Build history of the part. All positions in model axes, mm. Coordinates: 2 decimals unless noted, no trailing zeros. Order: outer loops, then holes, each group sorted by start corner. A loop starts at its lowest first (then second) coordinate and runs counter-clockwise, first axis right, second up. Notation, with made-up numbers: (11.5, 22) - (60.5, 22) arc R15 ccw to (60.5, 47) - close; hole circle Ø3 at (35, 9). An arc over 180 degrees is marked (long way). One line per item, written item: value.
from build123d import *

# Parameters (mm, degrees)
MODEL_R         = 1.5
MODEL_R_2       = 3.25
MODEL_R_3       = 1.25
EXTRUDE_1_DEPTH = 1


with BuildPart() as part:
    # Model → Бобышка-Вытянуть1 (new body)
    with BuildSketch(Plane.XY):
        with BuildLine():
            Line((-28.5, -69), (28.5, -69))
            ThreePointArc((28.5, -69), (29.207106781, -68.707106781), (29.5, -68))
            Line((29.5, -68), (29.5, -61))
            ThreePointArc((29.5, -61), (29.792893219, -60.292893219), (30.5, -60))
            Line((30.5, -60), (39, -60))
            ThreePointArc((39, -60), (39.707106781, -59.707106781), (40, -59))
            Line((40, -59), (40, -55))
            Line((40, -55), (40, -51))
            ThreePointArc((40, -51), (39.707106781, -50.292893219), (39, -50))
            Line((39, -50), (30.5, -50))
            ThreePointArc((30.5, -50), (29.792893219, -49.707106781), (29.5, -49))
            Line((29.5, -49), (29.5, -11))
            ThreePointArc((29.5, -11), (29.792893219, -10.292893219), (30.5, -10))
            Line((30.5, -10), (39, -10))
            ThreePointArc((39, -10), (39.707106781, -9.707106781), (40, -9))
            Line((40, -9), (40, -5))
            Line((40, -5), (40, -1))
            ThreePointArc((40, -1), (39.707106781, -0.292893219), (39, 0))
            Line((39, 0), (30.5, 0))
            ThreePointArc((30.5, 0), (29.792893219, 0.292893219), (29.5, 1))
            Line((29.5, 1), (29.5, 18))
            ThreePointArc((29.5, 18), (29.207106781, 18.707106781), (28.5, 19))
            Line((28.5, 19), (-28.5, 19))
            ThreePointArc((-28.5, 19), (-29.207106781, 18.707106781), (-29.5, 18))
            Line((-29.5, 18), (-29.5, 1))
            ThreePointArc((-29.5, 1), (-29.792893219, 0.292893219), (-30.5, 0))
            Line((-30.5, 0), (-39, 0))
            ThreePointArc((-39, 0), (-39.707106781, -0.292893219), (-40, -1))
            Line((-40, -1), (-40, -5))
            Line((-40, -5), (-40, -9))
            Line((-40, -9), (-40, -52))
            Line((-40, -52), (-40, -55))
            Line((-40, -55), (-40, -59))
            ThreePointArc((-40, -59), (-39.707106781, -59.707106781), (-39, -60))
            Line((-39, -60), (-30.5, -60))
            ThreePointArc((-30.5, -60), (-29.792893219, -60.292893219), (-29.5, -61))
            Line((-29.5, -61), (-29.5, -68))
            ThreePointArc((-29.5, -68), (-29.207106781, -68.707106781), (-28.5, -69))
        make_face()
        with Locations((-35, -5)):
            Circle(MODEL_R, mode=Mode.SUBTRACT)
        with Locations((-35, -55)):
            Circle(MODEL_R, mode=Mode.SUBTRACT)
        with Locations((35, -5)):
            Circle(MODEL_R, mode=Mode.SUBTRACT)
        with Locations((35, -55)):
            Circle(MODEL_R, mode=Mode.SUBTRACT)
        with Locations((-34, -20.4)):
            Circle(MODEL_R_2, mode=Mode.SUBTRACT)
        with Locations((25.4, -36.7)):
            Circle(MODEL_R_3, mode=Mode.SUBTRACT)
        with Locations((0, -36.7)):
            Circle(MODEL_R_3, mode=Mode.SUBTRACT)
        with Locations((25.4, 14.1)):
            Circle(MODEL_R_3, mode=Mode.SUBTRACT)
        with Locations((0, 14.1)):
            Circle(MODEL_R_3, mode=Mode.SUBTRACT)
        with Locations((-25.4, -11.3)):
            Circle(MODEL_R_3, mode=Mode.SUBTRACT)
        with Locations((-25.4, -36.7)):
            Circle(MODEL_R_3, mode=Mode.SUBTRACT)
        with Locations((-25.4, 14.1)):
            Circle(MODEL_R_3, mode=Mode.SUBTRACT)
        with Locations((25.4, -11.3)):
            Circle(MODEL_R_3, mode=Mode.SUBTRACT)
        with BuildLine():
            Line((-2.3, -8), (-2.3, 10.8))
            ThreePointArc((-2.3, 10.8), (-2.592893219, 11.507106781), (-3.3, 11.8))
            Line((-3.3, 11.8), (-22.1, 11.8))
            ThreePointArc((-22.1, 11.8), (-22.807106781, 11.507106781), (-23.1, 10.8))
            Line((-23.1, 10.8), (-23.1, -8))
            ThreePointArc((-23.1, -8), (-22.807106781, -8.707106781), (-22.1, -9))
            Line((-22.1, -9), (-3.3, -9))
            ThreePointArc((-3.3, -9), (-2.592893219, -8.707106781), (-2.3, -8))
        make_face(mode=Mode.SUBTRACT)
        with BuildLine():
            Line((2.3, -8), (2.3, 10.8))
            ThreePointArc((2.3, 10.8), (2.592893219, 11.507106781), (3.3, 11.8))
            Line((3.3, 11.8), (22.1, 11.8))
            ThreePointArc((22.1, 11.8), (22.807106781, 11.507106781), (23.1, 10.8))
            Line((23.1, 10.8), (23.1, -8))
            ThreePointArc((23.1, -8), (22.807106781, -8.707106781), (22.1, -9))
            Line((22.1, -9), (3.3, -9))
            ThreePointArc((3.3, -9), (2.592893219, -8.707106781), (2.3, -8))
        make_face(mode=Mode.SUBTRACT)
        with BuildLine():
            Line((-2.3, -14.6), (-2.3, -33.4))
            ThreePointArc((-2.3, -33.4), (-2.592893219, -34.107106781), (-3.3, -34.4))
            Line((-3.3, -34.4), (-22.1, -34.4))
            ThreePointArc((-22.1, -34.4), (-22.807106781, -34.107106781), (-23.1, -33.4))
            Line((-23.1, -33.4), (-23.1, -14.6))
            ThreePointArc((-23.1, -14.6), (-22.807106781, -13.892893219), (-22.1, -13.6))
            Line((-22.1, -13.6), (-3.3, -13.6))
            ThreePointArc((-3.3, -13.6), (-2.592893219, -13.892893219), (-2.3, -14.6))
        make_face(mode=Mode.SUBTRACT)
        with BuildLine():
            Line((2.3, -14.6), (2.3, -33.4))
            ThreePointArc((2.3, -33.4), (2.592893219, -34.107106781), (3.3, -34.4))
            Line((3.3, -34.4), (22.1, -34.4))
            ThreePointArc((22.1, -34.4), (22.807106781, -34.107106781), (23.1, -33.4))
            Line((23.1, -33.4), (23.1, -14.6))
            ThreePointArc((23.1, -14.6), (22.807106781, -13.892893219), (22.1, -13.6))
            Line((22.1, -13.6), (3.3, -13.6))
            ThreePointArc((3.3, -13.6), (2.592893219, -13.892893219), (2.3, -14.6))
        make_face(mode=Mode.SUBTRACT)
    extrude(amount=EXTRUDE_1_DEPTH)


solid = part.part
1. Two-plate mould, pull along X, no slides. Class faces 1 (the face through (25.24, -35.46, 0.49)), 2 (the face through (-1, -34, 1)): pulls with the +X half, pulls with the -X half, needs draft (parallel to the pull), parting line crosses it, or undercut.
Values found:
face 1: undercut
face 2: needs draft
2. Band-saw the part on D-D, the plane y = -5. Give the cut face in (x, z).
Values found:
outline: (-40, 0) - (-36.5, 0) - (-36.5, 1) - (-40, 1) - close; (-33.5, 0) - (-23.1, 0) - (-23.1, 1) - (-33.5, 1) - close; (-2.3, 0) - (2.3, 0) - (2.3, 1) - (-2.3, 1) - close; (23.1, 0) - (33.5, 0) - (33.5, 1) - (23.1, 1) - close; (36.5, 0) - (40, 0) - (40, 1) - (36.5, 1) - close
3. Band-saw the part on C-C, the plane x = 14. Give the cut face in (y, z), and give its area (3 significant figures).
Values found:
outline: (-69, 0) - (-34.4, 0) - (-34.4, 1) - (-69, 1) - close; (-13.6, 0) - (-9, 0) - (-9, 1) - (-13.6, 1) - close; (11.8, 0) - (19, 0) - (19, 1) - (11.8, 1) - close
area: 46.4 mm2
4. Probe line 1 along X through (y, z) = (-7, 0.2); line 2 along X through (y, z) = (3.5, 0.65); line 3 along Y through (x, z) = (-15, 0.4). List the from-to ranges inside material, lowest first.
Values found:
line 1: x = -40 to -23.1, -2.3 to 2.3, 23.1 to 40
line 2: x = -29.5 to -23.1, -2.3 to 2.3, 23.1 to 29.5
line 3: y = -69 to -34.4, -13.6 to -9, 11.8 to 19
5. Band-saw the part on A-A, the plane y = -36.7. Give the cut face in (x, z).
Values found:
outline: (-40, 0) - (-26.65, 0) - (-26.65, 1) - (-40, 1) - close; (-24.15, 0) - (-1.25, 0) - (-1.25, 1) - (-24.15, 1) - close; (1.25, 0) - (24.15, 0) - (24.15, 1) - (1.25, 1) - close; (26.65, 0) - (29.5, 0) - (29.5, 1) - (26.65, 1) - close
6. Band-saw the part on B-B, the plane x = 25.4. Give the cut face in (y, z).
Values found:
outline: (-69, 0) - (-37.95, 0) - (-37.95, 1) - (-69, 1) - close; (-35.45, 0) - (-12.55, 0) - (-12.55, 1) - (-35.45, 1) - close; (-10.05, 0) - (12.85, 0) - (12.85, 1) - (-10.05, 1) - close; (15.35, 0) - (19, 0) - (19, 1) - (15.35, 1) - close
7. Flat gauge pins, fed straight in: P1, Ø0.5, axis at x = 33, z = 0.5, coming from the +Y side; P2, Ø0.5, axis at y = -66, z = 0.5, coming from the -X side; P3, Ø1.8, axis at x = -35, y = -55, coming from the +Z side. Where does each tip first touch, or does it go through?
Values found:
P1: stops at y = 0
P2: stops at x = -29.5
P3: passes through
